The model under review builds one solid part; all positions refer to its coordinate system, in mm. A direction names the side the tool comes from. Round coordinates to 2 decimals unless told otherwise and drop trailing zeros. Loops run counter-clockwise (first coordinate to the right, second up) from the corner with the lowest first, then second, coordinate; pieces in that order, holes last. Notation, with made-up numbers: (17.5, -20) -> (32.5, -20) arc R36 cw to (32.5, 18) -> close; hole circle Ø6 at (61.5, -3). An arc over 180 degrees is marked (long way). Use a Markdown table: item, result. Add a question column.
1) Insertion check: pin 1 (1 mm diameter, centred on y = 30, z = -4.5, fed in from +X); pin 2 (2 mm diameter, centred on x = -85.5, z = -2, fed in from +Y); pin 3 (1 mm diameter, centred on x = -90.5, z = -4, fed in from -Y). Each pin has a flat end and moves straight along its axis. Give the tip position at first contact, or say it passes through.
2) Consider section B-B on y = 52. Give the boundary of the cut face in (x, z).
3) Mouldability with a two-part tool opening along Y and no side actions: class faces 3 (the cylindrical face through (-66.4, -5.8, -2.5)), 4 (the cylindrical face through (-52.588, 47.757, -2.535)), 5 (the flat face through (-50.73, 21.34, -2.46)), 6 (the cylindrical face through (-124.774, 14.4, -2.465)) as released by +Y, released by -Y, zero draft, split by the parting line, or undercut.
4) Consider section D-D on y = 44.5. Give the boundary of the cut face in (x, z).
5) For faces 1 (the flat face through (-81.218, 24.894, -2.465)), 2 (the flat face through (-93.345, -2.884, -2.465)), list the 3-axis set-ups (+Z, -Z, +X, -X, +Y, -Y) from which the entire face can be reached by the end or side of a thin tool; tool diameter is ignored.
6) Consider section C-C on z = -2.7. Give the boundary of the cut face in (x, y).
7) Consider section A-A on x = -71.5. Give the boundary of the cut face in (y, z).
8) Wall thickness on probe 1 along X at (y, z) = (52.5, -1.55); probe 2 along X at (y, z) = (29, -4.45); probe 3 along Y at (x, z) = (-85.5, -1.7): over which ranges is each line inside the solid? List them lowest first.
from build123d import *

# Parameters (mm, degrees)
BOSS_EXTRU_1_DEPTH           = 5
ENL_V_MAT_EXTRU_1_DEPTH      = 139.023902146
ENL_V_MAT_EXTRU_1_DEPTH_BACK = 139.023902146
ESQUISSE2_R                  = 3


with BuildPart() as part:
    # Esquisse1 → Boss.-Extru.1 (new body)
    with BuildSketch(Plane.XY):
        with BuildLine():
            Line((-56.676061624, -5.615526744), (-44.613461935, 49.069879799))
            ThreePointArc((-44.613461935, 49.069879799), (-47.521267958, 56.747400855), (-55.720555636, 57.161341672))
            Line((-55.720555636, 57.161341672), (-115.960936395, 19.676937291))
            ThreePointArc((-115.960936395, 19.676937291), (-124.816589866, 14.245466781), (-119.749865766, 5.176190229))
            Line((-119.749865766, 5.176190229), (-66.18965615, -11.173242359))
            ThreePointArc((-66.18965615, -11.173242359), (-60.216844676, -10.475935129), (-56.676061624, -5.615526744))
        make_face()
        Polygon((-62.953169806, 35.564136013), (-69.575176268, 5.543483348), (-98.978129472, 14.518832861), align=None, mode=Mode.SUBTRACT)
    extrude(amount=-BOSS_EXTRU_1_DEPTH)

    # Esquisse2 → Enlèv. mat.-Extru.1 (cut, two sides: drawn at the far end of the back side and taken through both)
    with BuildSketch(Plane.XY.offset(-ENL_V_MAT_EXTRU_1_DEPTH_BACK)):
        with Locations((-117.560209615, 12.349432588)):
            Circle(ESQUISSE2_R)
        with Locations((-64, -4)):
            Circle(ESQUISSE2_R)
        with Locations((-51.937400312, 50.685406543)):
            Circle(ESQUISSE2_R)
    extrude(amount=ENL_V_MAT_EXTRU_1_DEPTH + ENL_V_MAT_EXTRU_1_DEPTH_BACK, mode=Mode.SUBTRACT)


solid = part.part
Result set:
| question | item | result |
|---|---|---|
| 1 | pin 1 | x = -48.71 |
| 1 | pin 2 | y = 39.25 |
| 1 | pin 3 | y = -3.91 |
| 2 | outline | (-64.02, -5) -> (-54.63, -5) -> (-54.63, 0) -> (-64.02, 0) -> close; (-49.24, -5) -> (-44.55, -5) -> (-44.55, 0) -> (-49.24, 0) -> close |
| 3 | face 3 | undercut |
| 3 | face 4 | undercut |
| 3 | face 5 | released by -Y |
| 3 | face 6 | split by the parting line |
| 4 | outline | (-76.07, -5) -> (-45.62, -5) -> (-45.62, 0) -> (-76.07, 0) -> close |
| 5 | face 1 | +Z, -Z |
| 5 | face 2 | +Z, -Z, -X, -Y |
| 6 | outline | (-119.75, 5.18) -> (-66.19, -11.17) arc R7.5 ccw to (-56.68, -5.62) -> (-44.61, 49.07) arc R7.5 ccw to (-55.72, 57.16) -> (-115.96, 19.68) arc R7.5 ccw to start; hole circle Ø6 at (-117.56, 12.35); hole (-98.98, 14.52) -> (-69.58, 5.54) -> (-62.95, 35.56) -> close; hole circle Ø6 at (-64, -4); hole circle Ø6 at (-51.94, 50.69) |
| 7 | outline | (-9.55, -5) -> (6.13, -5) -> (6.13, 0) -> (-9.55, 0) -> close; (30.57, -5) -> (47.34, -5) -> (47.34, 0) -> (30.57, 0) -> close |
| 8 | probe 1 | -63.21 to -54.33, -49.55 to -44.66 |
| 8 | probe 2 | -100.98 to -74.19, -64.4 to -49.04 |
| 8 | probe 3 | -5.28 to 10.4, 22.39 to 38.63 |
